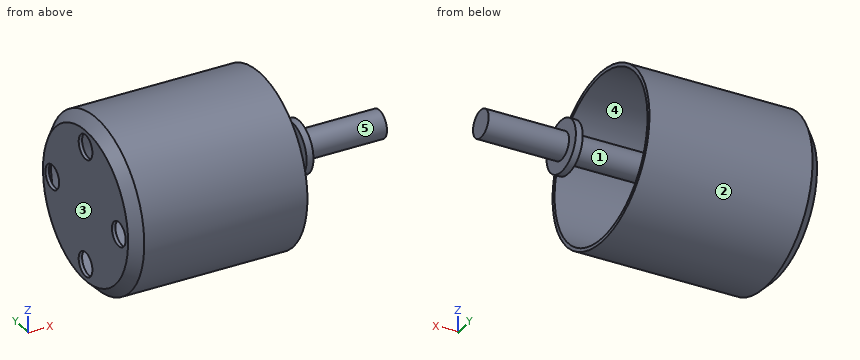
```python
from build123d import *

# Parameters (mm, degrees)
SKETCH2_R           = 4
BOSS_EXTRUDE1_DEPTH = 85.5
SKETCH3_R           = 3.5
CUT_EXTRUDE1_DEPTH  = 93.387093254
SKETCH4_R           = 7.5
BOSS_EXTRUDE2_DEPTH = 2


with BuildPart() as part:
    # Sketch1 → Revolve1 (revolve)
    with BuildSketch(Plane.XY, mode=Mode.PRIVATE) as revolve1_sk:
        Polygon((0, 21.75), (3, 24.75), (50.5, 24.75), (50.5, 23.75), (3.414213562, 23.75), (1, 21.335786438), (1, 0), (0, 0), align=None)
    revolve(revolve1_sk.sketch.rotate(Axis((0, 0, 0), (1, 0, 0)), 90), axis=Axis((0, 0, 0), (1, 0, 0)))

    # Sketch2 → Boss-Extrude1 (add)
    with BuildSketch(Plane(origin=(0, 0, 0), x_dir=(0, 0, -1), z_dir=(1, 0, 0))):
        with Locations(Location((0, 0, 0), (0, 0, 180))):
            Circle(SKETCH2_R)
    extrude(amount=BOSS_EXTRUDE1_DEPTH)

    # Sketch3 → Cut-Extrude1 (cut, through all)
    with BuildSketch(Plane.ZY):
        with Locations((0, 17)):
            Circle(SKETCH3_R)
        with Locations((17, 0)):
            Circle(SKETCH3_R)
        with Locations((0, -17)):
            Circle(SKETCH3_R)
        with Locations((-17, 0)):
            Circle(SKETCH3_R)
    extrude(amount=-CUT_EXTRUDE1_DEPTH, mode=Mode.SUBTRACT)

    # Sketch4 → Boss-Extrude2 (add)
    with BuildSketch(Plane(origin=(60.1, 0, 0), x_dir=(0, 0, -1), z_dir=(1, 0, 0))):
        Circle(SKETCH4_R)
    extrude(amount=BOSS_EXTRUDE2_DEPTH)


solid = part.part
```
Here's how the part is built. I have some questions about the finished solid (model axes, mm). Face numbers are marked on the shaded views. A direction names the side the tool comes from. Coordinates: 2 decimals unless noted, no trailing zeros. Write each loop counter-clockwise with the first axis right and the second up, starting at its lowest first coordinate (ties: lowest second). Pieces come first, ordered by that corner, then holes. Notation, with made-up numbers: (46.5, 34.5) - (54.5, 34.5) arc R13 cw to (54.5, 58.5) - close; hole circle Ø2 at (-35.75, 74). An arc over 180 degrees is marked (long way). One line per item, written item: value.
1) I need wall thicknesses on line 1 along Y through (x, z) = (32, 0); line 2 along X through (y, z) = (-12, 11); line 3 along Z through (x, y) = (36.5, 7.5). Which ranges of each line are inside material? Lowest first, please.
Model answer:
line 1: y = -24.75 to -23.75, -4 to 4, 23.75 to 24.75
line 2: x = 0 to 1
line 3: z = -23.59 to -22.53, 22.53 to 23.59
2) I'm going to push flat-ended pins straight in: P1, Ø5, axis at x = 18, z = 1, coming from the +Y side; P2, Ø1.5, axis at y = 4, z = -14.5, coming from the +X side; P3, Ø1.5, axis at x = 65, z = 1.5, coming from the +Y side. Where does each tip first touch, or does it pass through?
Model answer:
P1: stops at y = 24.75
P2: stops at x = 1
P3: stops at y = 3.93
3) We'd pull the mould along Z, two halves only. Please class the marked faces 3, 4 and 5: pulls with the +Z half, pulls with the -Z half, needs draft (parallel to the pull), parting line crosses it, or undercut.
Model answer:
face 3: needs draft
face 4: undercut
face 5: parting line crosses it
4) Suppose I cut it at B-B on x = 16. Write out the boundary of the cut face in (y, z), and give its area (3 significant figures).
Model answer:
outline: circle Ø49.5 at (0, 0); circle Ø8 at (0, 0); hole circle Ø47.5 at (0, 0)
area: 203 mm²
5) Suppose I cut it at A-A on y = 0. State how many separate pieces and enclosed holes the cut face has, and give its area (3 significant figures).
Model answer:
separate pieces: 3
enclosed holes: 0
area: 821 mm²
6) On a 3-axis mill with a long thin cutter (end or side, diameter ignored), from which of +Z, -Z, +X, -X, +Y, -Y can I reach the whole of each face in a straight line? I mean the marked faces 1 and 2. Say none if no direction works.
Model answer:
face 1: none
face 2: +X, -X
7) Suppose I cut it at C-C on x = 51.5. Write out the boundary of the cut face in (y, z), and give its area (3 significant figures).
Model answer:
outline: circle Ø8 at (0, 0)
area: 50.3 mm²
